from build123d import *

# Parameters (mm, degrees)
F0_R        = 0.8001
F1_DEPTH    = 6.1595
F2_R        = 0.762
F3_SIZE2    = 0.4399409051
F3_SIZE     = 0.254
F3_2_SIZE2  = 0.4399409051
F3_2_SIZE   = 0.254
F4_SIZE2    = 0.4399409051
F4_SIZE     = 0.254
F6_DEPTH    = 2.286
F8_R        = 0.508
F9_T1_DEPTH = 32.4811466943
F11_DEPTH   = 12.7


# Not quite as in the source:
# - a fillet or chamfer that OpenCascade refuses, or shapes differently, is made with other operations: its cross-section is extruded or revolved along the edge and cut away or added


with BuildPart() as f1:
    # F0 (on Right) → F1 (new body, symmetric)
    with BuildSketch(Plane.YZ):
        with BuildLine():
            Line((-19.6694904986, 1.6002), (-19.4160437172, 0))
            Line((-19.4160437172, 0), (19.4160437172, 0))
            Line((19.4160437172, 0), (19.2309873372, 1.1684))
            Line((19.2309873372, 1.1684), (15.8541987451, 1.1684))
            ThreePointArc((15.8541987451, 1.1684), (14.6580511896, 3.2349867583), (12.9176425998, 1.6002))
            Line((12.9176425998, 1.6002), (-5.7365591714, 1.6002))
            ThreePointArc((-5.7365591714, 1.6002), (-7.2552582858, 3.2512), (-8.7739574002, 1.6002))
            Line((-8.7739574002, 1.6002), (-19.6694904986, 1.6002))
        make_face()
        with Locations((-7.2552582858, 1.7272)):
            Circle(F0_R, mode=Mode.SUBTRACT)
        with Locations((14.4363417142, 1.7272)):
            Circle(F0_R, mode=Mode.SUBTRACT)
    extrude(amount=F1_DEPTH, both=True)

    # F2
    f2_edges = [f1.edges().sort_by_distance(p)[0] for p in [
        (0, -8.773957, 1.6002),
        (0, -5.736559, 1.6002),
        (0, 12.917643, 1.6002),
        (0, 15.854199, 1.1684),
    ]]
    fillet(f2_edges, radius=F2_R)

    # F3
    f3_edges = [f1.edges().sort_by_distance(p)[0] for p in [
        (6.1595, -8.055358, 1.7272),
        (-6.1595, -8.055358, 1.7272),
    ]]
    f3_side = f1.faces().sort_by_distance((0, -8.055358, 1.7272))[0]
    chamfer(f3_edges, length=F3_SIZE, length2=F3_SIZE2, reference=f3_side)

    # F3#2
    f3_2_edges = [f1.edges().sort_by_distance(p)[0] for p in [
        (6.1595, 13.636242, 1.7272),
    ]]
    f3_2_side = f1.faces().sort_by_distance((0, 13.636242, 1.7272))[0]
    chamfer(f3_2_edges, length=F3_2_SIZE, length2=F3_2_SIZE2, reference=f3_2_side)

    # F4
    f4_edges = [f1.edges().sort_by_distance(p)[0] for p in [
        (-6.1595, 13.636242, 1.7272),
    ]]
    f4_side = f1.faces().sort_by_distance((-0.127, 13.636242, 1.7272))[0]
    chamfer(f4_edges, length=F4_SIZE, length2=F4_SIZE2, reference=f4_side)

    # F5 (on Right) → F6 (cut, symmetric)
    with BuildSketch(Plane.YZ):
        with BuildLine():
            Line((-1.4272936791, 3.7511704683), (-13.4970735674, 4.5248900073))
            ThreePointArc((-13.4970735674, 4.5248900073), (-7.6939820902, 0.5220475291), (-1.4272936791, 3.7511704683))
        make_face()
        with BuildLine():
            Line((20.2263604549, 3.6906977019), (8.6020119823, 3.7614527913))
            ThreePointArc((8.6020119823, 3.7614527913), (14.3945992101, 0.508127038), (20.2263604549, 3.6906977019))
        make_face()
    extrude(amount=F6_DEPTH, both=True, mode=Mode.SUBTRACT)

    # F8
    f8_edges = [f1.edges().sort_by_distance(p)[0] for p in [
        (6.1595, 19.323516, 0.5842),
        (-6.1595, 19.323516, 0.5842),
    ]]
    fillet(f8_edges, radius=F8_R)

    # F9: fillet of radius 6.1722 on 2 edges, made by hand

    # F9_s2 → F9_t1 (cut)
    with BuildSketch(Plane(origin=(0, -3.1424532039, 19.8406686756), x_dir=(1, 0, 0), z_dir=(0, 0.156434465, -0.9876883406))):
        with BuildLine():
            ThreePointArc((6.1595, 13.0048), (4.3517044748, 17.3692044748), (-0.0127, 19.177))
            Line((-0.0127, 19.177), (6.1595, 19.177))
            Line((6.1595, 19.177), (6.1595, 13.0048))
        make_face()
        with BuildLine():
            ThreePointArc((0.0127, 19.177), (-4.3517044748, 17.3692044748), (-6.1595, 13.0048))
            Line((-6.1595, 13.0048), (-6.1595, 19.177))
            Line((-6.1595, 19.177), (0.0127, 19.177))
        make_face()
    extrude(amount=F9_T1_DEPTH, mode=Mode.SUBTRACT)

    # F10 (on line) → F11 (cut, symmetric)
    with BuildSketch(Plane(origin=(0, -0.4444158842, 2.8059314619), x_dir=(1, 0, 0), z_dir=(0, -0.156434465, 0.9876883406))):
        Polygon((5.9055, -9.7789869341), (6.1595, -9.7789869341), (6.1595, -8.338481352), align=None)
        Polygon((-6.1595, -8.338481352), (-6.1595, -9.7789869341), (-5.9055, -9.7789869341), align=None)
    extrude(amount=F11_DEPTH, both=True, mode=Mode.SUBTRACT)


solid = f1.part
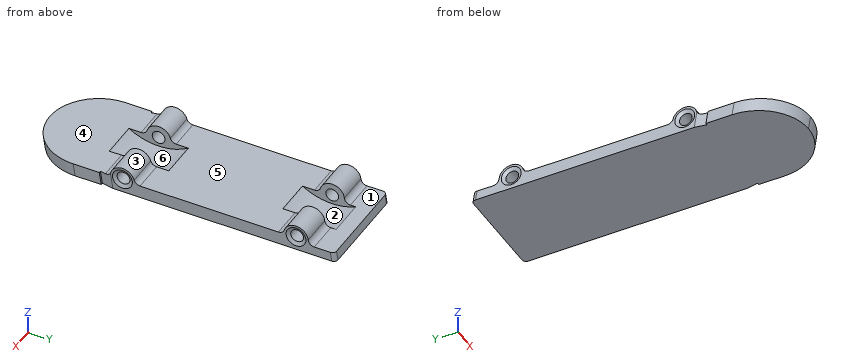
Model file for the job. Use its own axes, mm. Face numbers are marked on the shaded views. A direction names the side the tool comes from. Coordinates: 2 decimals unless noted, no trailing zeros. Write each loop counter-clockwise with the first axis right and the second up, starting at its lowest first coordinate (ties: lowest second). Pieces come first, ordered by that corner, then holes. Notation, with made-up numbers: (-22, -33) - (-1, -33) arc R16 cw to (-1, -28) - close; hole circle Ø3 at (-5, 2.25). An arc over 180 degrees is marked (long way). Write each question's results on one line, items separated by ' | '. Start each with the question number.
1) Cut at B-B (y = 2). Write the cut outline in (x, z), then the cut area to 3 significant figures.
2) Cut at A-A (x = -3.5). Write the cut outline in (y, z), then the cut area to 3 significant figures.
3) Cut at D-D (y = 11.5). Write the cut outline in (x, z), then the cut area to 3 significant figures.
4) Flat gauge pins, fed straight in: P1, Ø1.4, axis at y = -7.26, z = 1.73, coming from the +X side; P2, Ø1.5, axis at x = 3, y = -8.5, coming from the +Z side; P3, Ø6, axis at x = -1.5, y = 1.5, coming from the +Z side; P4, Ø0.8, axis at x = -2.5, y = 18, coming from the +Z side. Where does each tip first touch, or does it go through?
5) Mould opens along Y. For the marked faces 1, 2 and 3 say: pulls with the +Y half, pulls with the -Y half, needs draft (parallel to the pull), parting line crosses it, or undercut.
6) 3-axis set-ups, long thin cutter, end or side, ignore diameter. For the marked faces 4, 5 and 6: which of +Z, -Z, +X, -X, +Y, -Y reach the whole face in a straight line?
7) Cut at C-C (x = 1). Write the cut outline in (y, z), then the cut area to 3 significant figures.
8) Probe line 1 along Y through (x, z) = (-5.25, 1.75); line 2 along Y through (x, z) = (-4, 1.05); line 3 along Z through (x, y) = (5, 4.5). List the from-to ranges inside material, lowest first. Write a range as from..to.
Returned:
1) outline: (-6.16, 0) - (6.16, 0) - (6.16, 1.6) - (-6.16, 1.6) - close | area: 19.7 mm^2
2) outline: (-18.56, 1.6) - (-18.31, 0) - (19.42, 0) - (19.23, 1.17) - (16.71, 1.17) arc R0.76 cw to (15.95, 1.86) arc R1.52 ccw to (12.97, 2.15) arc R0.76 cw to (12.24, 1.6) - (-5.06, 1.6) arc R0.76 cw to (-5.79, 2.15) arc R1.52 ccw to (-8.72, 2.15) arc R0.76 cw to (-9.45, 1.6) - close; hole circle Ø1.6 at (-7.26, 1.73); hole circle Ø1.6 at (14.44, 1.73) | area: 63.4 mm^2
3) outline: (-6.16, 0) - (6.16, 0) - (6.16, 1.6) - (2.29, 1.6) - (2.29, 1.17) - (-2.29, 1.17) - (-2.29, 1.6) - (-6.16, 1.6) - close | area: 17.7 mm^2
4) P1: through | P2: z = 3.17 | P3: z = 1.6 | P4: z = 1.17
5) face 1: needs draft | face 2: undercut | face 3: undercut
6) face 4: +Z, +X, -X, -Y | face 5: +Z, +X, -X | face 6: +Z
7) outline: (-19.58, 1.6) - (-19.33, 0) - (19.42, 0) - (19.23, 1.17) - (17.37, 1.17) arc R6.86 cw to (10.72, 1.6) - (-3.54, 1.6) arc R6.86 cw to (-10.97, 1.6) - close | area: 50.4 mm^2
8) line 1: -9..-8.06, -6.46..-5.51, 12.69..13.64, 15.24..15.97 | line 2: -18.08..-7.68, -6.83..14.01, 14.86..19.25 | line 3: 0..1.6
